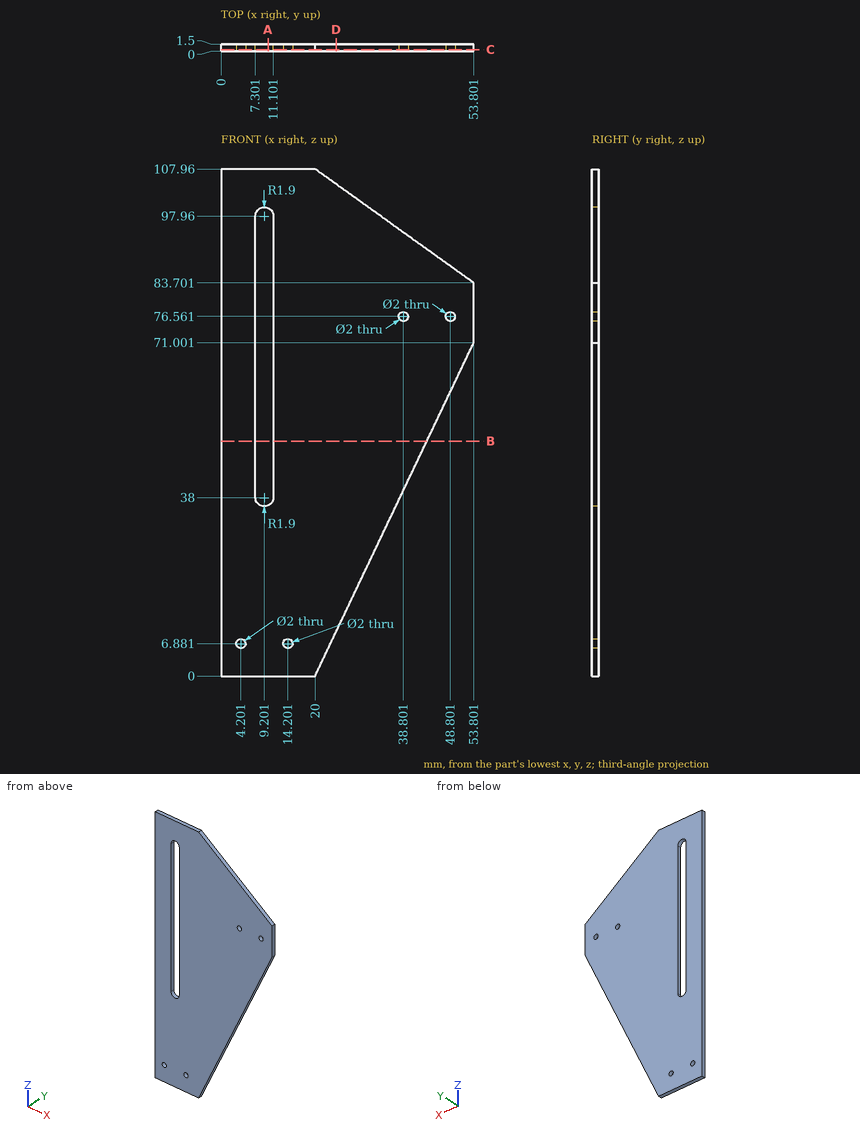
Part print with two shaded views. Sizes in mm from the minimum x, y, z corner. Give positions to 0.01 mm unless a question says otherwise; leave off trailing zeros. Loops run counter-clockwise (first coordinate to the right, second up) from the corner with the lowest first, then second, coordinate; pieces in that order, holes last. Notation, with made-up numbers: (33.5, -12) - (62.5, -12) arc R24 cw to (62.5, 8) - close; hole circle Ø6 at (-0.75, -37). An arc over 180 degrees is marked (long way). Put each result on its own line as item: value.
Q1. Slice it at D-D (x = 24.5). Give the cut face in (y, z).
Filled in:
outline: (0, 9.45) - (1.5, 9.45) - (1.5, 104.73) - (0, 104.73) - close
Q2. Slice it at B-B (z = 50). Give the cut face in (x, y).
Filled in:
outline: (0, 0) - (7.3, 0) - (7.3, 1.5) - (0, 1.5) - close; (11.1, 0) - (43.8, 0) - (43.8, 1.5) - (11.1, 1.5) - close
Q3. Flat gauge pins, fed straight in: pin 1 (1.8 mm diameter, centred on x = 4.2, z = 6.88, fed in from -Y); pin 2 (3 mm diameter, centred on x = 13.5, z = 21.5, fed in from -Y). Where does each tip first touch, or does it go through?
Filled in:
pin 1: passes through
pin 2: stops at y = 0
Q4. Probe line 1 along X through (y, z) = (1.25, 72.5); line 2 along X through (y, z) = (1, 77); line 3 along X through (y, z) = (0.4, 7.5) (1 decimal). List the from-to ranges inside material, lowest first.
Filled in:
line 1: x = 0 to 7.3, 11.1 to 53.8
line 2: x = 0 to 7.3, 11.1 to 37.9, 39.7 to 47.9, 49.7 to 53.8
line 3: x = 0 to 3.4, 5 to 13.4, 15 to 23.6
Q5. Slice it at A-A (x = 10). Give the cut face in (y, z).
Filled in:
outline: (0, 0) - (1.5, 0) - (1.5, 36.28) - (0, 36.28) - close; (0, 99.68) - (1.5, 99.68) - (1.5, 107.96) - (0, 107.96) - close
Q6. Slice it at C-C (y = 0.3). Give the cut face in (x, z), plus the area to 3 significant figures.
Filled in:
outline: (0, 0) - (20, 0) - (53.8, 71) - (53.8, 83.7) - (20, 107.96) - (0, 107.96) - close; hole circle Ø2 at (4.2, 6.88); hole (7.3, 38) arc R1.9 ccw to (11.1, 38) - (11.1, 97.96) arc R1.9 ccw to (7.3, 97.96) - close; hole circle Ø2 at (14.2, 6.88); hole circle Ø2 at (38.8, 76.56); hole circle Ø2 at (48.8, 76.56)
area: 3,950 mm²
